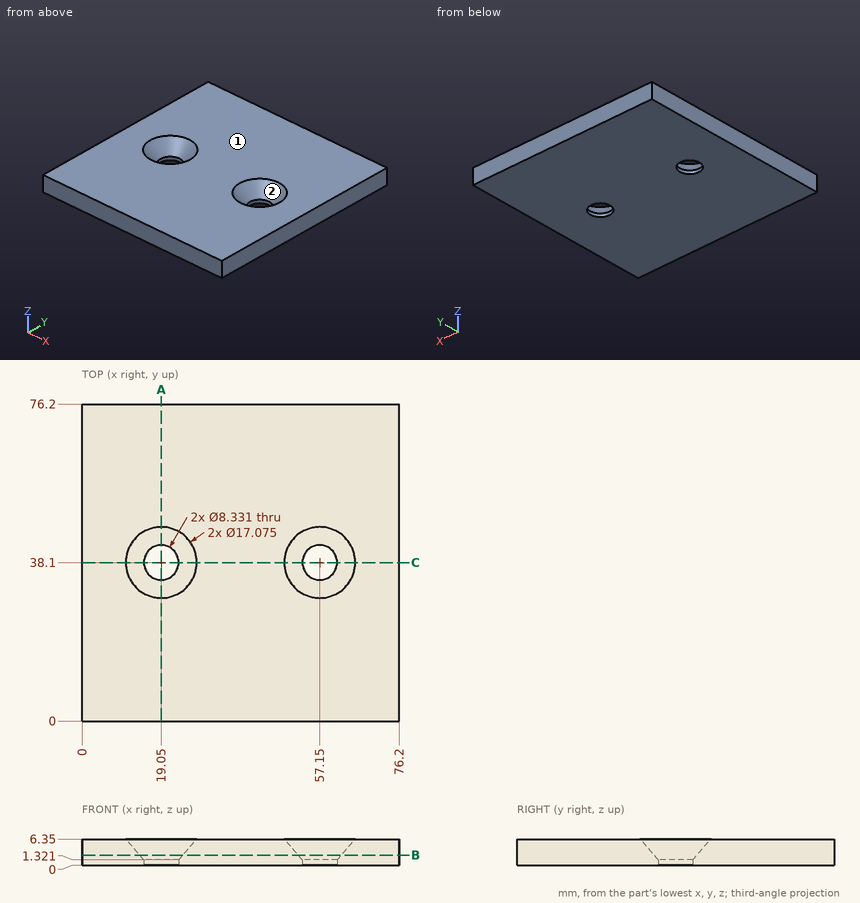
Answer from the drawing. Dimensions are ordinates in mm from the lowest x, y and z of the part. Give positions to 0.01 mm unless a question says otherwise; leave off trailing zeros. Write each loop counter-clockwise with the first axis right and the second up, starting at its lowest first coordinate (ties: lowest second). Pieces come first, ordered by that corner, then holes. Notation, with made-up numbers: (47, 69) - (95, 69) arc R32 cw to (95, 106) - close; hole circle Ø8 at (-18, 39). An arc over 180 degrees is marked (long way). Answer in a Markdown table with one row per item. Add a question column.
Item 1: Section C-C, the plane y = 38.1 is taken. Count the separate pieces of the cut face and the enclosed holes in it, and give its area (3 significant figures).
Item 2: Section B-B, the plane z = 2.5 is taken. Write down the section's boundary in (x, y).
Item 3: A flat-ended cylindrical pin translates along its axis: P1, Ø5, axis at x = 19.05, y = 38.1, coming from the +Z side. Find the tip coordinate at first contact, or state that the pin passes through.
Item 4: Section A-A, the plane x = 19.05 is taken. Write down the section's boundary in (y, z).
Item 5: Find the intervals of material crossed by L1, parallel to Y at x = 19.05, z = 0.45; L2, parallel to X at y = 38.5, z = 4.5; L3, parallel to Z at x = 59, y = 45, in increasing order.
Item 6: Determine the mould class of the marked faces 1 and 2 for opening direction X: pulls with the +X half, pulls with the -X half, needs draft (parallel to the pull), parting line crosses it, or undercut.
Recorded:
| question | item | result |
|---|---|---|
| 1 | separate pieces | 3 |
| 1 | enclosed holes | 0 |
| 1 | area | 334 mm2 |
| 2 | outline | (0, 0) - (76.2, 0) - (76.2, 76.2) - (0, 76.2) - close; hole circle Ø10.38 at (19.05, 38.1); hole circle Ø10.38 at (57.15, 38.1) |
| 3 | P1 | passes through |
| 4 | outline | (0, 0) - (33.93, 0) - (33.93, 1.32) - (29.56, 6.35) - (0, 6.35) - close; (42.27, 0) - (76.2, 0) - (76.2, 6.35) - (46.64, 6.35) - (42.27, 1.32) - close |
| 5 | L1 | y = 0 to 33.93, 42.27 to 76.2 |
| 5 | L2 | x = 0 to 12.13, 25.97 to 50.23, 64.07 to 76.2 |
| 5 | L3 | z = 0 to 4.75 |
| 6 | face 1 | needs draft |
| 6 | face 2 | undercut |
